from build123d import *

# Parameters (mm, degrees)
REVOLVE1_ANGLE           = 180
SKETCH3_W                = 69.85
SKETCH3_H                = 25.4
SKETCH3_W_2              = 50.8
SKETCH3_H_2              = 6.35
BOSS_EXTRUDE7_DEPTH      = 25.4
BOSS_EXTRUDE7_DEPTH_BACK = 38.1


with BuildPart() as part:
    # Sketch2 → Revolve1 (revolve)
    with BuildSketch(Plane(origin=(0, 0, 0), x_dir=(1, 0, 0), z_dir=(0, 1, 0))):
        with BuildLine():
            Line((32.496202247, -75.759218491), (32.496202247, -102.830579492))
            add(Edge.make_bspline(
                [(82.058028303, 7.870345482), (93.041481389, 34.162455024), (112.348086196, -13.725828539), (106.284293116, -68.651897164), (61.355001648, -101.966794635), (32.496202247, -102.830579492)],
                knots=[0, 0, 0, 0, 0.26758911, 0.512711999, 1, 1, 1, 1], degree=3))
            ThreePointArc((82.058028303, 7.870345482), (70.916457376, -42.027591177), (32.496202247, -75.759218491))
        make_face()
    revolve(axis=Axis((32.496202247, 0, 75.759218491), (0, 0, 1)), revolution_arc=REVOLVE1_ANGLE)

    # Sketch3 → Boss-Extrude7 (add, two sides)
    with BuildSketch(Plane(origin=(32.496202247, 0, 102.830579492), x_dir=(0.999552356, 0, 0.029918022), z_dir=(-0.029918022, 0, 0.999552356))) as boss_extrude7_sk:
        with Locations((1.700295248, 31.70443969)):
            Rectangle(SKETCH3_W, SKETCH3_H)
        with Locations((1.700295248, 31.70443969)):
            Rectangle(SKETCH3_W_2, SKETCH3_H_2, mode=Mode.SUBTRACT)
    extrude(amount=BOSS_EXTRUDE7_DEPTH)
    extrude(boss_extrude7_sk.sketch, amount=-BOSS_EXTRUDE7_DEPTH_BACK)


solid = part.part
Input: part model. Units: mm. Frame: model coordinates. Coordinates: 2 decimals unless noted, no trailing zeros. Order: outer loops, then holes, each group sorted by start corner. A loop starts at its lowest first (then second) coordinate and runs counter-clockwise, first axis right, second up. Notation, with made-up numbers: M 56.5,76 L 96.5,76 A20 ccw 96.5,99 Z; hole C -34,-19.75 d11. An arc over 180 degrees is marked long. Answer in a Markdown table with one row per item.
(1) Contact query for flat-ended pins moving along their axis: pin 1 Ø2 at (x, z) = (14, 45.5) entering from -Y; pin 2 Ø8 at (y, z) = (25.5, 106.5) entering from +X; pin 3 Ø3 at (y, z) = (63, 15.5) entering from -X; pin 4 Ø20.5 at (x, z) = (51.5, 99) entering from -Y. Output: stop coordinate, or through.
Numbers:
| item | result |
|---|---|
| pin 1 | stops at y = 30.17 |
| pin 2 | stops at x = 69.15 |
| pin 3 | stops at x = -11.33 |
| pin 4 | stops at y = 0 |
(2) Material intervals for line 1 (Y direction, x = 50.5, z = 116.5); line 2 (X direction, y = 23, z = -4); line 3 (X direction, y = 5, z = 58.5), sorted ascending. Write a range as [from, to].
Numbers:
| item | result |
|---|---|
| line 1 | y = [19, 28.53], [34.88, 44.4] |
| line 2 | x = [-34.34, -11.72], [76.71, 99.34] |
| line 3 | x = [-36.02, 7.41], [57.59, 101.02] |
(3) Section query A-A, the plane z = 115.5. Output: boundary loops of the cut face in (x, y).
Numbers:
| item | result |
|---|---|
| outline | M -1.12,19 L 68.76,19 L 68.76,44.4 L -1.12,44.4 Z; hole M 8.41,28.53 L 59.23,28.53 L 59.23,34.88 L 8.41,34.88 Z |
